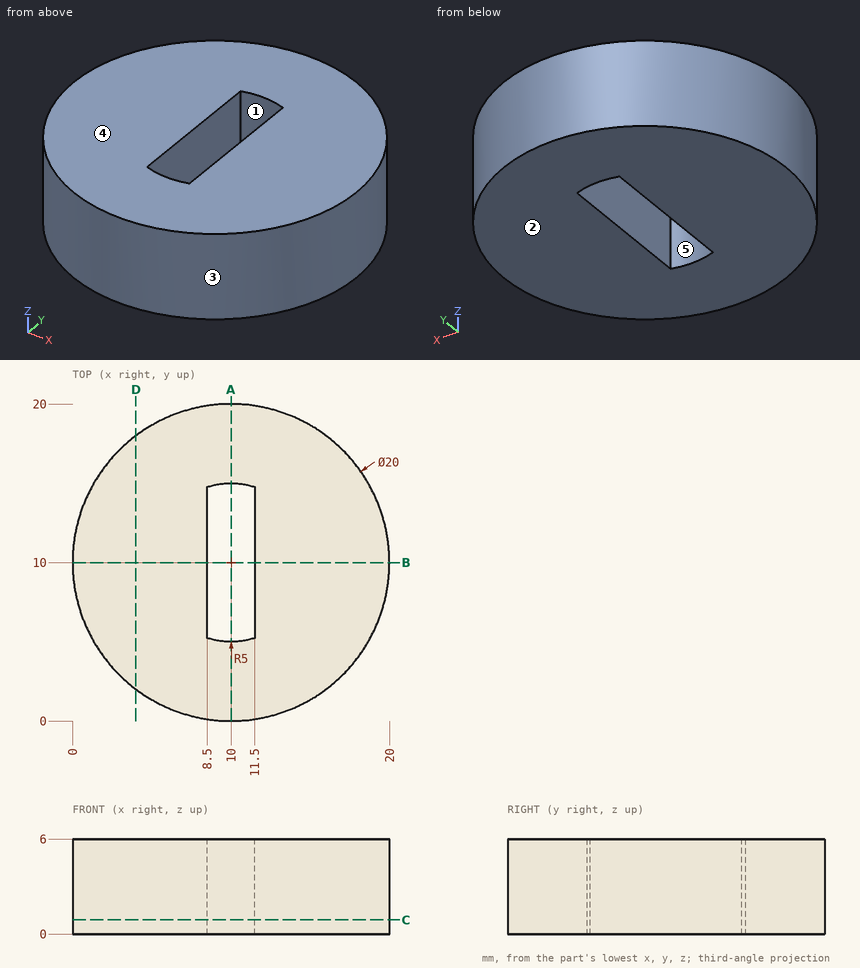
Geometry check sheet. Reference: drawing and pictorial views, mm from the part's lowest x, y, z. A direction names the side the tool comes from. Give positions to 0.01 mm unless a question says otherwise; leave off trailing zeros. Write each loop counter-clockwise with the first axis right and the second up, starting at its lowest first coordinate (ties: lowest second). Pieces come first, ordered by that corner, then holes. Notation, with made-up numbers: (-0.75, -6.5) -> (20.25, -6.5) arc R22 ccw to (20.25, 15.5) -> close; hole circle Ø8 at (61, -30.5). An arc over 180 degrees is marked (long way). One line per question, with ' | ' between items.
Item 1: Depth check by flat-ended pin: pin 1 (2 mm diameter, centred on x = 12.5, z = 0.5, fed in from -Y); pin 2 (1.5 mm diameter, centred on x = 12.5, z = 1, fed in from +Y); pin 3 (1 mm diameter, centred on x = 5.5, z = 1.5, fed in from -Y). Enter the tip coordinate at first touch or a pass-through.
Determined:
pin 1: y = 0.11 | pin 2: y = 19.85 | pin 3: y = 0.83
Item 2: Sectioned sample at D-D, the plane x = 4. Record the boundary of the cut face in (y, z), plus the area to 3 significant figures.
Determined:
outline: (2, 0) -> (18, 0) -> (18, 6) -> (2, 6) -> close | area: 96.0 mm^2
Item 3: Scan lines: line 1 along X through (y, z) = (12.5, 3.6); line 2 along X through (y, z) = (12, 5.2); line 3 along X through (y, z) = (3.5, 4.3). Record each from-to range of solid material in increasing order.
Determined:
line 1: 0.32 to 8.5, 11.5 to 19.68 | line 2: 0.2 to 8.5, 11.5 to 19.8 | line 3: 2.4 to 17.6
Item 4: Sectioned sample at B-B, the plane y = 10. Record the boundary of the cut face in (x, z), plus the area to 3 significant figures.
Determined:
outline: (0, 0) -> (8.5, 0) -> (8.5, 6) -> (0, 6) -> close; (11.5, 0) -> (20, 0) -> (20, 6) -> (11.5, 6) -> close | area: 102 mm^2
Item 5: Sectioned sample at C-C, the plane z = 0.9. Record the boundary of the cut face in (x, y), plus the area to 3 significant figures.
Determined:
outline: circle Ø20 at (10, 10); hole (8.5, 5.23) arc R5 ccw to (11.5, 5.23) -> (11.5, 14.77) arc R5 ccw to (8.5, 14.77) -> close | area: 285 mm^2
Item 6: Draft check along X on the marked faces 3, 4 and 5. Enter one of: released by +X, released by -X, zero draft, split by the parting line, or undercut.
Determined:
face 3: split by the parting line | face 4: zero draft | face 5: undercut
Item 7: Access from +Z, -Z, +X, -X, +Y, -Y to the whole of each face (thin tool, end or side, straight path). Record for the marked faces 1 and 2.
Determined:
face 1: +Z, -Z | face 2: -Z, +X, -X, +Y, -Y
Item 8: Sectioned sample at A-A, the plane x = 10. Record the boundary of the cut face in (y, z).
Determined:
outline: (0, 0) -> (5, 0) -> (5, 6) -> (0, 6) -> close; (15, 0) -> (20, 0) -> (20, 6) -> (15, 6) -> close
